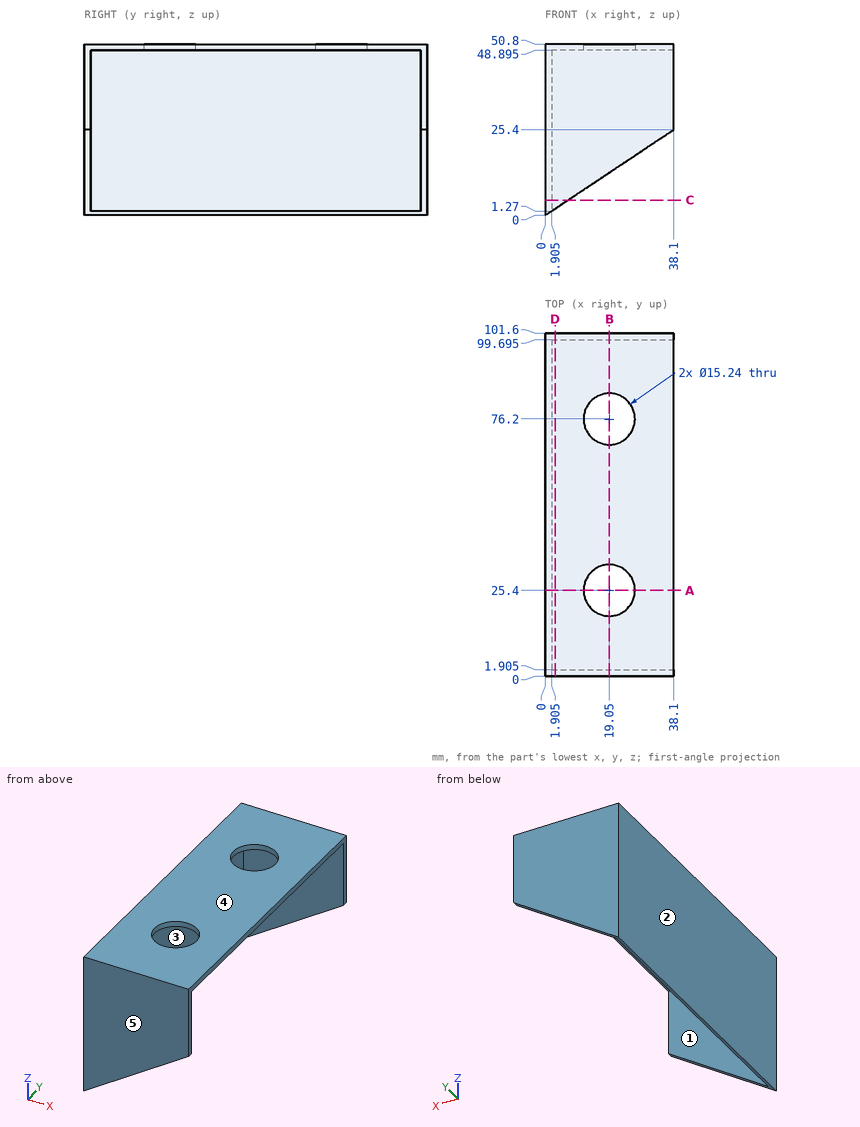
Study the drawing (mm; zero at the part's minimum x, y, z) and answer. A direction names the side the tool comes from. Give positions to 0.01 mm unless a question says otherwise; leave off trailing zeros. Order: outer loops, then holes, each group sorted by start corner. A loop starts at its lowest first (then second) coordinate and runs counter-clockwise, first axis right, second up.
1) Find section B-B on x = 19.05. Write down the section's boundary in (y, z) (3 decimals).
Reported:
outline: (0, 12.7) - (1.905, 12.7) - (1.905, 48.895) - (17.78, 48.895) - (17.78, 50.8) - (0, 50.8) - close; (33.02, 48.895) - (68.58, 48.895) - (68.58, 50.8) - (33.02, 50.8) - close; (83.82, 48.895) - (99.695, 48.895) - (99.695, 12.7) - (101.6, 12.7) - (101.6, 50.8) - (83.82, 50.8) - close
2) Find section A-A on y = 25.4. Write down the section's boundary in (x, z) (3 decimals).
Reported:
outline: (0, 0) - (1.905, 1.27) - (1.905, 48.895) - (11.43, 48.895) - (11.43, 50.8) - (0, 50.8) - close; (26.67, 48.895) - (38.1, 48.895) - (38.1, 50.8) - (26.67, 50.8) - close
3) Find section C-C on z = 4.5. Write down the section's boundary in (x, y) (3 decimals), then the cut area to 3 significant figures.
Reported:
outline: (0, 0) - (6.75, 0) - (6.75, 1.905) - (1.905, 1.905) - (1.905, 99.695) - (6.75, 99.695) - (6.75, 101.6) - (0, 101.6) - close
area: 212 mm2
4) Determine the mould class of the marked faces 3, 4 and 5 for opening direction Y: pulls with the +Y half, pulls with the -Y half, needs draft (parallel to the pull), parting line crosses it, or undercut.
Reported:
face 3: undercut
face 4: needs draft
face 5: pulls with the -Y half
5) Given P1, Ø18, axis at x = 26.5, z = 30.5, coming from the -Y side; P2, Ø17.5, axis at x = 19.05, y = 76.2, coming from the -Z side (3 decimals); P3, Ø2, axis at y = 59.5, z = 17.5, coming from the +X side (3 decimals), each flat-ended and moving along its own axis, determine where each tip first touches the part or whether it passes through.
Reported:
P1: stops at y = 0
P2: stops at z = 48.895
P3: stops at x = 1.905
6) Find section D-D on x = 3. Write down the section's boundary in (y, z) (3 decimals).
Reported:
outline: (0, 2) - (1.905, 2) - (1.905, 48.895) - (99.695, 48.895) - (99.695, 2) - (101.6, 2) - (101.6, 50.8) - (0, 50.8) - close
7) Consider line 1 along Y through (x, z) = (19, 50); line 2 along X through (y, z) = (76, 49); line 3 along X through (y, z) = (9, 7.5) (3 decimals). Determine where each line is inside the solid, lowest interval first.
Reported:
line 1: y = 0 to 17.78, 33.02 to 68.58, 83.82 to 101.6
line 2: x = 0 to 11.43, 26.67 to 38.1
line 3: x = 0 to 1.905
8) For the marked faces 1 and 2, determine the directions among +Z, -Z, +X, -X, +Y, -Y from which every point of the face is accessible in a straight line to the end or side of a thin tool.
Reported:
face 1: -Z, +X
face 2: +Z, -Z, -X, +Y, -Y
